```python
from build123d import *

# Parameters (mm, degrees)
SKETCH_1_R               = 150
EXTRUDE_1_DEPTH          = 5
SKETCH_2_R               = 20
EXTRUDE_2_DEPTH          = 100
PATTERN_CIRCULAR_1_COUNT = 3
SKETCH_3_R               = 2.5
EXTRUDE_3_DEPTH          = 15


with BuildPart() as part:
    # 草图1 → 凸台-拉伸1 (new body)
    with BuildSketch(Plane(origin=(0, 0, 0), x_dir=(1, 0, 0), z_dir=(0, 1, 0))):
        with Locations(Location((0, 0, 0), (0, 0, 270))):
            Circle(SKETCH_1_R)
    extrude(amount=EXTRUDE_1_DEPTH)

    # 草图2 → 凸台-拉伸2 (add)
    with BuildSketch(Plane(origin=(0, 5, 0), x_dir=(1, 0, 0), z_dir=(0, 1, 0))):
        with Locations(Location((0, -120, 0), (0, 0, 270))):
            Circle(SKETCH_2_R)
    extrude_2 = extrude(amount=EXTRUDE_2_DEPTH)

    # 阵列(圆周)1: 凸台-拉伸2 ×3 about axis
    pattern_circular_1_axis = Axis((0, 0, 0), (0, 1, 0))
    for i in range(1, PATTERN_CIRCULAR_1_COUNT):
        add(extrude_2.rotate(pattern_circular_1_axis, i * 360 / PATTERN_CIRCULAR_1_COUNT))

    # 草图3 → 凸台-拉伸3 (add)
    with BuildSketch(Plane.XZ):
        with Locations(Location((0, 0, 0), (0, 0, 90))):
            Circle(SKETCH_3_R)
    extrude(amount=EXTRUDE_3_DEPTH)


solid = part.part
```
The listing builds one solid part. Answer for the finished solid, in the listing's coordinates (mm). A direction names the side the tool comes from. Give positions to 0.01 mm unless a question says otherwise; leave off trailing zeros. Order: outer loops, then holes, each group sorted by start corner. A loop starts at its lowest first (then second) coordinate and runs counter-clockwise, first axis right, second up.
1) Find section B-B on x = 27. Write down the section's boundary in (y, z), then the cut area to 3 significant figures.
Reported:
outline: (0, -147.55) - (5, -147.55) - (5, 147.55) - (0, 147.55) - close
area: 1,480 mm2
2) Find section C-C on y = 48.5. Write down the section's boundary in (x, z).
Reported:
outline: circle Ø40 at (-103.92, -60); circle Ø40 at (0, 120); circle Ø40 at (103.92, -60)
3) Find section D-D on z = -60. Write down the section's boundary in (x, y).
Reported:
outline: (-137.48, 0) - (137.48, 0) - (137.48, 5) - (123.92, 5) - (123.92, 105) - (83.92, 105) - (83.92, 5) - (-83.92, 5) - (-83.92, 105) - (-123.92, 105) - (-123.92, 5) - (-137.48, 5) - close
4) For faces 1 (the face through (0.88, 54.3, 100.02)), 2 (the face through (104, 105, -60)), determine the directions among +Z, -Z, +X, -X, +Y, -Y from which every point of the face is accessible in a straight line to the end or side of a thin tool.
Reported:
face 1: +Y
face 2: +Z, -Z, +X, -X, +Y
5) Find section A-A on z = 120. Write down the section's boundary in (x, y).
Reported:
outline: (-90, 0) - (90, 0) - (90, 5) - (20, 5) - (20, 105) - (-20, 105) - (-20, 5) - (-90, 5) - close
6) Consider line 1 along X through (y, z) = (75.5, -59.5); line 2 along Y through (x, z) = (67, 51); line 3 along Y through (x, z) = (0, 104). Determine where each line is inside the solid, lowest interval first.
Reported:
line 1: x = -123.92 to -83.93, 83.93 to 123.92
line 2: y = 0 to 5
line 3: y = 0 to 105
7) Determine the mould class of faces 3 (the face through (120.79, 54.3, -49.25)), 4 (the face through (-91.273, 2.465, -119.035)), 5 (the face through (2, 0, -2)) for opening direction X: pulls with the +X half, pulls with the -X half, needs draft (parallel to the pull), parting line crosses it, or undercut.
Reported:
face 3: undercut
face 4: parting line crosses it
face 5: needs draft
8) Given P1, Ø3, axis at y = 78, z = 113, coming from the +X side; P2, Ø8, axis at x = 17, z = 40, coming from the -Y side; P3, Ø4, axis at x = 83.5, y = 25, coming from the +Z side; P4, Ø10, axis at x = -28, y = 79, coming from the -Z side, each flat-ended and moving along its own axis, determine where each tip first touches the part or whether it passes through.
Reported:
P1: stops at x = 19.23
P2: stops at y = 0
P3: stops at z = -52.22
P4: passes through
